For this review, use the dimensioned drawing (mm, ordinates from the lowest corner) and the shaded views. Give positions to 0.01 mm unless a question says otherwise; leave off trailing zeros. Write each loop counter-clockwise with the first axis right and the second up, starting at its lowest first coordinate (ties: lowest second). Pieces come first, ordered by that corner, then holes.
1) We need section C-C on x = 40. Give the boundary of the cut face in (y, z), and give its area (3 significant figures).
2) We need section B-B on z = 15. Give the boundary of the cut face in (x, y), and give its area (3 significant figures).
3) Wall thickness on line 1 along Z through (x, y) = (40, 1.2); line 2 along X through (y, z) = (0.75, 15); line 3 along X through (y, z) = (1.3, 6): over which ranges is each line inside the solid? List them lowest first.
4) We need section A-A on y = 0.8. Give the boundary of the cut face in (x, z), and give its area (3 significant figures).
5) For P1, Ø3.5, axis at x = 40, z = 6, coming from the +Y side, flat-tipped, find the tip position at first contact; note if it passes through.
6) We need section D-D on x = 12. Give the boundary of the cut face in (y, z).
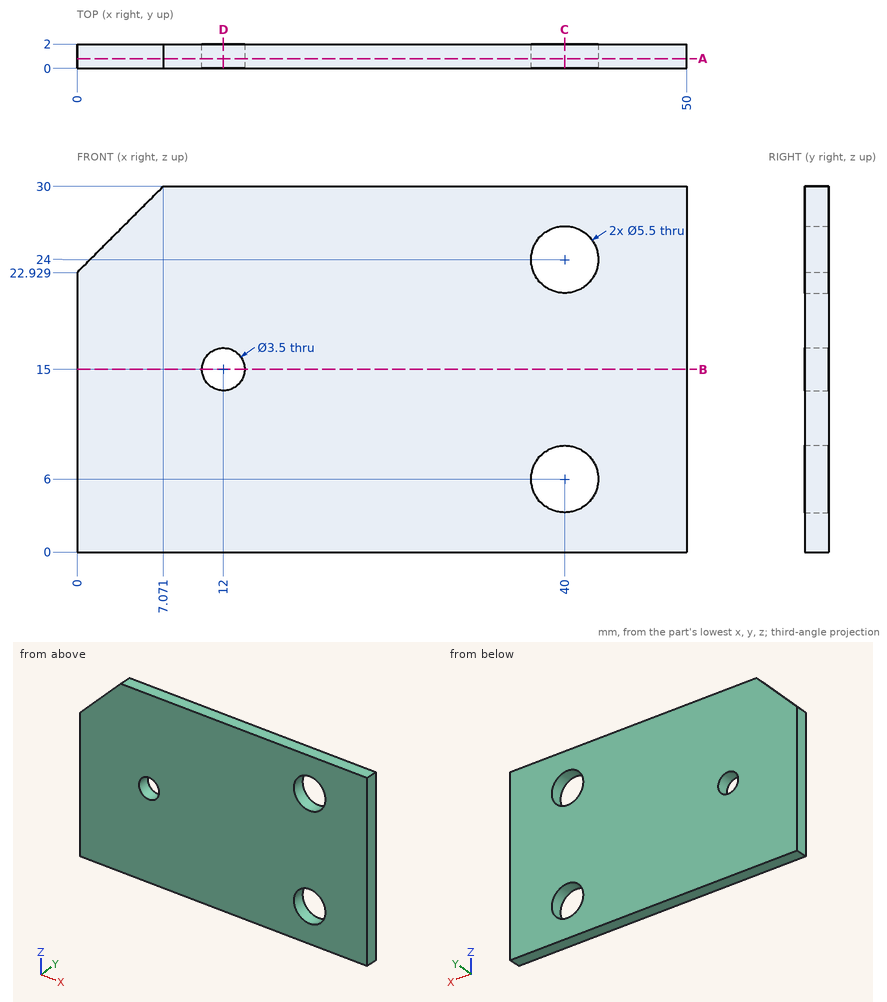
Results list:
1. outline: (0, 0) - (2, 0) - (2, 3.25) - (0, 3.25) - close; (0, 8.75) - (2, 8.75) - (2, 21.25) - (0, 21.25) - close; (0, 26.75) - (2, 26.75) - (2, 30) - (0, 30) - close
1. area: 38.0 mm2
2. outline: (0, 0) - (10.25, 0) - (10.25, 2) - (0, 2) - close; (13.75, 0) - (50, 0) - (50, 2) - (13.75, 2) - close
2. area: 93.0 mm2
3. line 1: z = 0 to 3.25, 8.75 to 21.25, 26.75 to 30
3. line 2: x = 0 to 10.25, 13.75 to 50
3. line 3: x = 0 to 37.25, 42.75 to 50
4. outline: (0, 0) - (50, 0) - (50, 30) - (7.07, 30) - (0, 22.93) - close; hole circle Ø3.5 at (12, 15); hole circle Ø5.5 at (40, 6); hole circle Ø5.5 at (40, 24)
4. area: 1,420 mm2
5. P1: passes through
6. outline: (0, 0) - (2, 0) - (2, 13.25) - (0, 13.25) - close; (0, 16.75) - (2, 16.75) - (2, 30) - (0, 30) - close
